Here's how the part is built. I have some questions about the finished solid (model axes, mm). Face numbers are marked on the shaded views. A direction names the side the tool comes from. Round coordinates to 2 decimals unless told otherwise and drop trailing zeros. Write each loop counter-clockwise with the first axis right and the second up, starting at its lowest first coordinate (ties: lowest second). Pieces come first, ordered by that corner, then holes. Notation, with made-up numbers: (83, 37) -> (95, 37) arc R25 cw to (95, 49) -> close; hole circle Ø4 at (87, -18). An arc over 180 degrees is marked (long way). Answer as CSV lines item,"result".
from build123d import *

# Parameters (mm, degrees)
P_IDAT_VYSUNUT_M1_DEPTH  = 60
ODEBRAT_VYSUNUT_M1_REACH = 130.841
P_IDAT_VYSUNUT_M2_DEPTH  = 10
M8_Z_VIT1_D              = 6.8
M8_Z_VIT1_CSINK_D        = 8.05
M8_Z_VIT1_CSINK_ANGLE    = 90
ZAOBLIT1_R               = 2
ZAOBLIT2_R               = 3
ZKOSEN_1_SIZE            = 3
ZKOSEN_1_SIZE2           = 1.091910703


# Read off the part's stored shape, not the designer's step: Přidat vysunutím3
with BuildPart() as part:
    # Skica1 → Přidat vysunutím1 (new body)
    with BuildSketch(Plane.XY):
        with BuildLine():
            Line((0, 0), (0, 10))
            Line((0, 10), (31.270166538, 10))
            ThreePointArc((31.270166538, 10), (75.040171699, 39.681187851), (110, 0))
            Line((110, 0), (100, 0))
            ThreePointArc((100, 0), (70, 30), (40, 0))
            Line((40, 0), (0, 0))
        make_face()
    extrude(amount=P_IDAT_VYSUNUT_M1_DEPTH)

    # Skica2 → Odebrat vysunutím1 (cut, up to next)
    with BuildSketch(Plane(origin=(0, 10, 0), x_dir=(1, 0, 0), z_dir=(0, 1, 0)), mode=Mode.PRIVATE) as odebrat_vysunut_m1_sk1:
        with BuildLine():
            Line((20, -20), (20, -50))
            ThreePointArc((20, -50), (15, -55), (10, -50))
            Line((10, -50), (10, -20))
            ThreePointArc((10, -20), (15, -15), (20, -20))
        make_face()
    odebrat_vysunut_m1_tool1 = extrude(odebrat_vysunut_m1_sk1.sketch, amount=-ODEBRAT_VYSUNUT_M1_REACH, mode=Mode.PRIVATE) & part.part
    add(odebrat_vysunut_m1_tool1.solids().sort_by_distance((15, 10, 35))[0], mode=Mode.SUBTRACT)

    # Skica3 → Přidat vysunutím2 (add)
    with BuildSketch(Plane(origin=(0, 0, 0), x_dir=(-1, 0, 0), z_dir=(0, 0, -1))):
        with BuildLine():
            Line((0, 0), (0, 20))
            ThreePointArc((0, 20), (-8.786796564, 41.213203436), (-30, 50))
            Line((-30, 50), (-90, 50))
            ThreePointArc((-90, 50), (-111.213203436, 41.213203436), (-120, 20))
            Line((-120, 20), (-120, 0))
            Line((-120, 0), (0, 0))
        make_face()
    extrude(amount=P_IDAT_VYSUNUT_M2_DEPTH)

    # Přidat vysunutím3 outline → Přidat vysunutím3 (revolve)
    with BuildSketch(Plane(origin=(70, 0, 35), x_dir=(1, 0, 0), z_dir=(0, 0, 1))):
        Polygon((7.5, 60), (0, 60), (0, 37.657552573), (13.486640745, 37.657552573), align=None)
    revolve(axis=Axis((70, 0, 35), (0, 1, 0)))

    # M8 závit1 (through all)
    with Locations(Plane(origin=(0, 60, 0), x_dir=(1, 0, 0), z_dir=(0, 1, 0))):
        with Locations((70, -35)):
            CounterSinkHole(M8_Z_VIT1_D / 2, M8_Z_VIT1_CSINK_D / 2, counter_sink_angle=M8_Z_VIT1_CSINK_ANGLE)

    # Zaoblit1
    zaoblit1_edges = [part.edges().sort_by_distance(p)[0] for p in [
        (31.270166538, 10, 30),
        (0, 5, 60),
        (15.635083269, 10, 0),
        (75.040171699, 39.681187851, 0),
    ]]
    fillet(zaoblit1_edges, radius=ZAOBLIT1_R)

    # Zaoblit2
    zaoblit2_edges = [part.edges().sort_by_distance(p)[0] for p in [
        (56.513435034, 37.657835378, 35.000000009),
        (70, 30, 0),
    ]]
    fillet(zaoblit2_edges, radius=ZAOBLIT2_R)

    # Zkosení1
    zkosen_1_edges = [part.edges().sort_by_distance(p)[0] for p in [
        (70, 30, 60),
    ]]
    zkosen_1_side = [part.faces().sort_by_distance(p)[0] for p in [
        (70, 30, 31.5),
    ]]
    chamfer(zkosen_1_edges, length=ZKOSEN_1_SIZE, length2=ZKOSEN_1_SIZE2, reference=zkosen_1_side[0])


solid = part.part
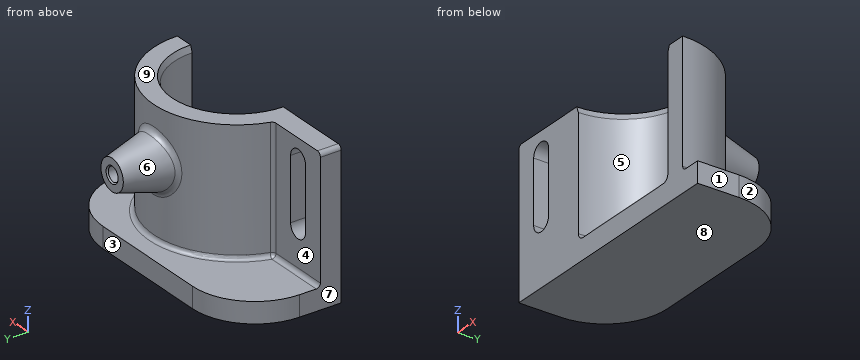
Item 1: I need wall thicknesses on L1, parallel to Z at x = 70, y = 37.25; L2, parallel to Z at x = 70, y = 46.75; L3, parallel to X at y = 6.5, z = 31.5. Which ranges of each line are inside material? Lowest first, please.
Results found:
L1,"z = -10 to 31.6, 38.4 to 60"
L2,"z = -10 to 0, 23.95 to 31.6, 38.4 to 46.05"
L3,"x = 0 to 10, 20 to 40.71, 99.29 to 109.47"
Item 2: Will these pins go through, and if not, where does the flat tip stop? pin 1 (5 mm diameter, centred on x = 74, z = -3, fed in from +Y); pin 2 (11 mm diameter, centred on y = 7, z = 39.5, fed in from +X); pin 3 (4 mm diameter, centred on y = 13.5, z = 6, fed in from -X); pin 4 (5.5 mm diameter, centred on x = 70, z = 35, fed in from -Y).
Results found:
pin 1,"stops at y = 50"
pin 2,"stops at x = 109.97"
pin 3,"stops at x = 31.69"
pin 4,"passes through"
Item 3: For the marked faces 1, 2, 3, 4 and 5, which set-ups out of +Z, -Z, +X, -X, +Y, -Y let a thin tool reach every point of the face, with its end or its side?
Results found:
face 1,"+Z, -Z, +X, +Y, -Y"
face 2,"+Z, -Z, +X, +Y"
face 3,"-Z, +X, -X, +Y"
face 4,"+Z, -X, +Y"
face 5,"+Z, -Y"
Item 4: If we mould it in two halves opening along Z, with no side actions, what happens to the marked faces 6, 7, 8 and 9? For each: pulls with the +Z half, pulls with the -Z half, needs draft (parallel to the pull), parting line crosses it, or undercut.
Results found:
face 6,"undercut"
face 7,"needs draft"
face 8,"pulls with the -Z half"
face 9,"pulls with the +Z half"
Item 5: Suppose I cut it at A-A, the plane x = 15.5. List the corners of the cut face in (y, z) for me.
Results found:
outline,"(0, -10) -> (46.26, -10) -> (46.26, 0) -> (12, 0) arc R2 cw to (10, 2) -> (10, 15.03) -> (0, 15.03) -> close; (0, 54.97) -> (10, 54.97) -> (10, 60) -> (0, 60) -> close"
Item 6: Suppose I cut it at B-B, the plane y = 45.5. List the corners of the cut face in (x, z) for me, then the cut area to 3 significant figures.
Results found:
outline,"(14.2, -10) -> (105.8, -10) -> (105.8, 0) -> (14.2, 0) -> close; circle Ø22.77 at (70, 35); hole circle Ø6.8 at (70, 35)"
area,"1,290 mm²"
